Input: part model. Units: mm. Frame: model coordinates. Give positions to 0.01 mm unless a question says otherwise; leave off trailing zeros. Write each loop counter-clockwise with the first axis right and the second up, starting at its lowest first coordinate (ties: lowest second). Pieces come first, ordered by that corner, then holes. Notation, with made-up numbers: (-7, 31) - (21, 31) arc R25 cw to (21, 48) - close; hole circle Ø5 at (65.25, -1). An arc over 180 degrees is marked (long way). Answer as CSV lines item,"result".
```python
from build123d import *

# Parameters (mm, degrees)
SKETCH_1_W          = 105
SKETCH_1_H          = 106
EXTRUDE_1_DEPTH     = 8
SKETCH_3_R          = 3.1
CUT_EXTRUDE_1_DEPTH = 10
SKETCH_5_R          = 7.5
EXTRUDE_2_DEPTH     = 90
FILLET_1_R          = 2


with BuildPart() as part:
    # 草图1 → 凸台-拉伸1 (new body)
    with BuildSketch(Plane(origin=(0, 0, 0), x_dir=(1, 0, 0), z_dir=(0, 1, 0))):
        with Locations((52.5, 53)):
            Rectangle(SKETCH_1_W, SKETCH_1_H)
    extrude(amount=EXTRUDE_1_DEPTH)

    # 草图3 → 切除-拉伸1 (cut)
    with BuildSketch(Plane(origin=(0, 8, 0), x_dir=(1, 0, 0), z_dir=(0, 1, 0))):
        with Locations(Location((90, 13, 0), (0, 0, 270))):
            Circle(SKETCH_3_R)
        with Locations(Location((90, 93, 0), (0, 0, 270))):
            Circle(SKETCH_3_R)
        with Locations(Location((10, 93, 0), (0, 0, 270))):
            Circle(SKETCH_3_R)
        with Locations(Location((10, 13, 0), (0, 0, 270))):
            Circle(SKETCH_3_R)
    extrude(amount=-CUT_EXTRUDE_1_DEPTH, mode=Mode.SUBTRACT)

    # 草图5 → 凸台-拉伸2 (add)
    with BuildSketch(Plane(origin=(0, 8, 0), x_dir=(1, 0, 0), z_dir=(0, 1, 0))):
        with Locations(Location((52.5, 53, 0), (0, 0, 90))):
            Circle(SKETCH_5_R)
    extrude(amount=EXTRUDE_2_DEPTH)

    # 圆角1
    fillet_1_edges = [part.edges().sort_by_distance(p)[0] for p in [
        (52.5, 8, -45.5),
        (52.5, 98, -45.5),
    ]]
    fillet(fillet_1_edges, radius=FILLET_1_R)


solid = part.part
```
Item 1: Cut plane A-A on z = -13. Return the cut outline in (x, y).
The answers:
outline,"(0, 0) - (6.9, 0) - (6.9, 8) - (0, 8) - close; (13.1, 0) - (86.9, 0) - (86.9, 8) - (13.1, 8) - close; (93.1, 0) - (105, 0) - (105, 8) - (93.1, 8) - close"
Item 2: Cut plane D-D on z = -67. Return the cut outline in (x, y).
The answers:
outline,"(0, 0) - (105, 0) - (105, 8) - (0, 8) - close"
Item 3: Cut plane B-B on x = 10. Return the cut outline in (y, z), plus the area to 3 significant figures.
The answers:
outline,"(0, -106) - (8, -106) - (8, -96.1) - (0, -96.1) - close; (0, -89.9) - (8, -89.9) - (8, -16.1) - (0, -16.1) - close; (0, -9.9) - (8, -9.9) - (8, 0) - (0, 0) - close"
area,"749 mm²"
Item 4: Contact query for flat-ended pins moving along their axis: pin 1 (1.5 mm diameter, centred on x = 78.5, z = -71, fed in from +Y); pin 2 (6 mm diameter, centred on x = 44, y = 18.5, fed in from -Z). Output: stop coordinate, or through.
The answers:
pin 1,"y = 8"
pin 2,"z = -58.1"
Item 5: Ray query, line 1 (X direction, y = 4.5, z = -13); line 2 (Y direction, x = 62.5, z = -18); line 3 (Z direction, x = 47, y = 29). Return the intervals inside material, ascending. Write a range as from..to.
The answers:
line 1,"0..6.9, 13.1..86.9, 93.1..105"
line 2,"0..8"
line 3,"-58.1..-47.9"
Item 6: Cut plane C-C on y = 13. Return the cut outline in (x, z), plus the area to 3 significant figures.
The answers:
outline,"circle Ø15 at (52.5, -53)"
area,"177 mm²"
Item 7: Mould query, pull axis Z, two halves, no side actions, for faces 1 (the face through (88.813, 4.056, -90.136)), 2 (the face through (52, 0, -54)), 3 (the face through (59.82, 52.4, -51.37)), 4 (the face through (52, 4, 0)). Classes: +Z half, -Z half, draft (parallel to the pull), parting line (faces both ways), or undercut.
The answers:
face 1,"undercut"
face 2,"draft"
face 3,"parting line"
face 4,"+Z half"
